Here's the drawing with two shaded views (mm, measured from the low corner). I have some questions. A direction names the side the tool comes from. Coordinates: 2 decimals unless noted, no trailing zeros. Loops run counter-clockwise (first coordinate to the right, second up) from the corner with the lowest first, then second, coordinate; pieces in that order, holes last.
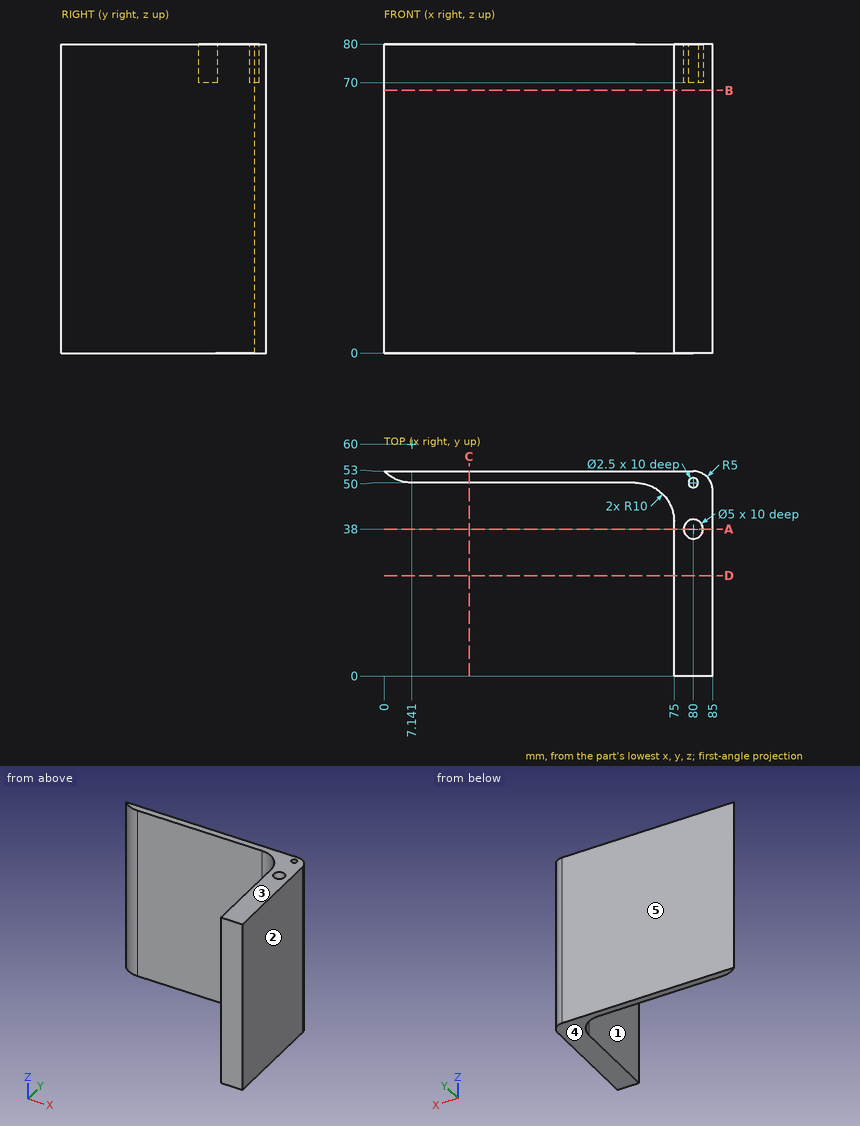
(1) I want a section at C-C on x = 22. Write out the boundary of the cut face in (y, z).
Check values:
outline: (50, 0) - (53, 0) - (53, 80) - (50, 80) - close
(2) I want a section at D-D on y = 26. Write out the boundary of the cut face in (x, z), then the cut area to 3 significant figures.
Check values:
outline: (75, 0) - (85, 0) - (85, 80) - (75, 80) - close
area: 800 mm2
(3) If we mould it in two halves opening along Z, with no side actions, what happens to the marked faces 3, 4 and 5? For each: released by +Z, released by -Z, zero draft, split by the parting line, or undercut.
Check values:
face 3: released by +Z
face 4: released by -Z
face 5: zero draft
(4) Which directions (+Z, -Z, +X, -X, +Y, -Y) give clear straight access to the entire face, cutting with the end or side of a thin tool? Please do the marked faces 1 and 2.
Check values:
face 1: +Z, -Z, -X, -Y
face 2: +Z, -Z, +X, +Y, -Y
(5) I want a section at B-B on z = 68. Write out the boundary of the cut face in (x, y).
Check values:
outline: (0, 53) arc R10 ccw to (7.14, 50) - (65, 50) arc R10 cw to (75, 40) - (75, 0) - (85, 0) - (85, 48) arc R5 ccw to (80, 53) - close
(6) I want a section at A-A on y = 38. Write out the boundary of the cut face in (x, z).
Check values:
outline: (75, 0) - (85, 0) - (85, 80) - (82.5, 80) - (82.5, 70) - (77.5, 70) - (77.5, 80) - (75, 80) - close
(7) If I drill on probe 1 along Y at (x, z) = (80, 76.5); probe 2 along X at (y, z) = (17, 14); probe 3 along Y at (x, z) = (53, 46), over which ranges is the centre line in solid material (lowest first)?
Check values:
probe 1: y = 0 to 35.5, 40.5 to 48.75, 51.25 to 53
probe 2: x = 75 to 85
probe 3: y = 50 to 53
(8) I'm going to push flat-ended pins straight in: pin 1 (3 mm diameter, centred on x = 59, z = 28.5, fed in from -Y); pin 2 (1.5 mm diameter, centred on y = 8, z = 35, fed in from -X). Where does each tip first touch, or does it pass through?
Check values:
pin 1: stops at y = 50
pin 2: stops at x = 75
